Build history of the part. All positions in model axes, mm. Face numbers are marked on the shaded views. A direction names the side the tool comes from. Give positions to 0.01 mm unless a question says otherwise; leave off trailing zeros. Order: outer loops, then holes, each group sorted by start corner. A loop starts at its lowest first (then second) coordinate and runs counter-clockwise, first axis right, second up. Notation, with made-up numbers: (-9, 53) - (18, 53) arc R26 ccw to (18, 89) - close; hole circle Ø2 at (37, -26.75). An arc over 180 degrees is marked (long way). Use a Markdown table: item, result. Add a question column.
(1) Which spindle directions (+Z, -Z, +X, -X, +Y, -Y) get a long thin tool onto all of the face, cutting with end or side? Do the marked faces 5, 6, 7 and 8. Say none if no direction does.
(2) Mould opens along X. For the marked faces 1, 2, 3 and 4 say: +X half, -X half, draft (parallel to the pull), parting line (faces both ways), or undercut.
(3) Flat gauge pins, fed straight in: pin 1 (9.5 mm diameter, centred on y = 7, z = 19.5, fed in from +X); pin 2 (8 mm diameter, centred on x = 14, y = 23.5, fed in from +Z); pin 3 (2 mm diameter, centred on x = 20.5, z = 24.5, fed in from +Y); pin 4 (10 mm diameter, centred on x = 16, z = 17.5, fed in from -Y). Where does each tip first touch, or does it go through?
(4) Slice it at B-B (z = 10). Write the cut outline in (x, y), then the cut area to 3 significant figures.
(5) Wall check: line 1 (Y direction, x = 15.25, z = 8); line 2 (X direction, y = 12.5, z = 20); line 3 (X direction, y = 26.5, z = 29). Give the ranges that are in metal, low to high.
(6) Slice it at A-A (y = 15). Write the cut outline in (x, z).
(7) Slice it at C-C (x = 12). Write the cut outline in (y, z).
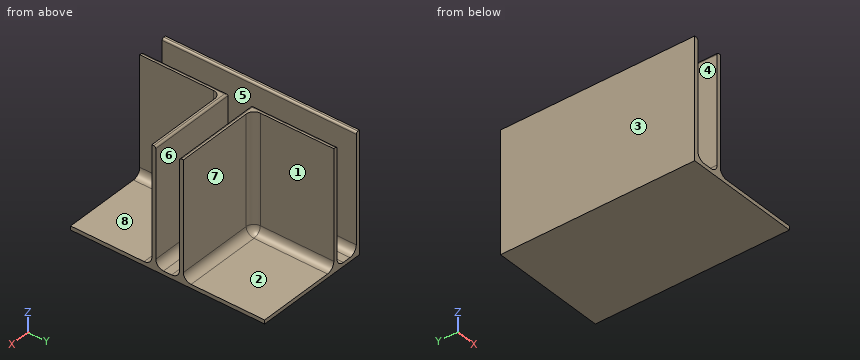
from build123d import *

# Parameters (mm, degrees)
SKETCH1_W           = 30
SKETCH1_H           = 50
BOSS_EXTRUDE1_DEPTH = 1
SKETCH2_W           = 1
SKETCH2_H           = 50
BOSS_EXTRUDE2_DEPTH = 30
FILLET4_R           = 2
FILLET5_R           = 0.5


with BuildPart() as part:
    # Sketch1 → Boss-Extrude1 (new body)
    with BuildSketch(Plane.XY):
        with Locations((15, 25)):
            Rectangle(SKETCH1_W, SKETCH1_H)
    extrude(amount=BOSS_EXTRUDE1_DEPTH)

    # Sketch2 → Boss-Extrude2 (add)
    with BuildSketch(Plane.XY.offset(1)):
        Polygon((7.1, 0), (8.1, 0), (8.1, 20.95), (30, 20.95), (30, 21.95), (8.1, 21.95), (7.1, 21.95), align=None)
        with Locations((0.5, 25)):
            Rectangle(SKETCH2_W, SKETCH2_H)
        Polygon((7.1, 50), (8.1, 50), (8.1, 29.05), (30, 29.05), (30, 28.05), (8.1, 28.05), (7.1, 28.05), align=None)
    extrude(amount=BOSS_EXTRUDE2_DEPTH)

    # Fillet4
    fillet4_edges = [part.edges().sort_by_distance(p)[0] for p in [
        (1, 25, 1),
        (7.1, 10.975, 1),
        (8.1, 10.475, 1),
        (19.05, 20.95, 1),
        (8.1, 20.95, 16),
        (18.55, 21.95, 1),
        (7.1, 39.025, 1),
        (18.55, 28.05, 1),
        (19.05, 29.05, 1),
        (8.1, 39.525, 1),
        (8.1, 29.05, 16),
    ]]
    fillet(fillet4_edges, radius=FILLET4_R)

    # Fillet5
    fillet5_edges = [part.edges().sort_by_distance(p)[0] for p in [
        (1, 25, 31),
        (7.1, 10.975, 31),
        (18.55, 21.95, 31),
        (7.1, 39.025, 31),
        (18.55, 28.05, 31),
    ]]
    fillet(fillet5_edges, radius=FILLET5_R)


solid = part.part
Solution:
| question | item | result |
|---|---|---|
| 1 | face 5 | +Z, +Y, -Y |
| 1 | face 6 | +Z, +X |
| 1 | face 7 | +Z, +X, +Y |
| 1 | face 8 | +Z, +X, -Y |
| 2 | face 1 | +X half |
| 2 | face 2 | draft |
| 2 | face 3 | -X half |
| 2 | face 4 | undercut |
| 3 | pin 1 | x = 8.1 |
| 3 | pin 2 | z = 31 |
| 3 | pin 3 | y = 29.05 |
| 3 | pin 4 | y = 20.95 |
| 4 | outline | (0, 0) - (1, 0) - (1, 50) - (0, 50) - close; (7.1, 0) - (8.1, 0) - (8.1, 18.95) arc R2 cw to (10.1, 20.95) - (30, 20.95) - (30, 21.95) - (7.1, 21.95) - close; (7.1, 28.05) - (30, 28.05) - (30, 29.05) - (10.1, 29.05) arc R2 cw to (8.1, 31.05) - (8.1, 50) - (7.1, 50) - close |
| 4 | area | 139 mm2 |
| 5 | line 1 | 20.95 to 21.95, 28.05 to 29.05 |
| 5 | line 2 | 0 to 1, 7.1 to 8.1 |
| 5 | line 3 | 0 to 1 |
| 6 | outline | (0, 0) - (30, 0) - (30, 1) - (10.1, 1) arc R2 cw to (8.1, 3) - (8.1, 31) - (7.6, 31) arc R0.5 ccw to (7.1, 30.5) - (7.1, 3) arc R2 cw to (5.1, 1) - (3, 1) arc R2 cw to (1, 3) - (1, 30.5) arc R0.5 ccw to (0.5, 31) - (0, 31) - close |
| 7 | outline | (0, 0) - (50, 0) - (50, 1) - (31.05, 1) arc R2 cw to (29.05, 3) - (29.05, 31) - (28.55, 31) arc R0.5 ccw to (28.05, 30.5) - (28.05, 3) arc R2 cw to (26.05, 1) - (23.95, 1) arc R2 cw to (21.95, 3) - (21.95, 30.5) arc R0.5 ccw to (21.45, 31) - (20.95, 31) - (20.95, 3) arc R2 cw to (18.95, 1) - (0, 1) - close |
